For this review, take the finished solid that the model builds, in its own axes (mm). A direction names the side the tool comes from. Coordinates: 2 decimals unless noted, no trailing zeros. Write each loop counter-clockwise with the first axis right and the second up, starting at its lowest first coordinate (ties: lowest second). Pieces come first, ordered by that corner, then holes.
1) Insertion check: P1, Ø2, axis at x = -11.5, z = -10.5, coming from the +Y side; P2, Ø10, axis at x = -7.5, y = 46.5, coming from the +Z side; P3, Ø9, axis at x = -10.5, z = 11, coming from the -Y side. Each pin has a flat end and moves straight along its axis. Give the tip position at first contact, or say it passes through.
2) Mouldability with a two-part tool opening along X and no side actions: class faces 1 (the face through (-6.55, 46.07, 5.19)), 2 (the face through (9, 10, 9)), 3 (the face through (-4, 0, -4)), 4 (the face through (15.244, 50.75, -2.002)) as pulls with the +X half, pulls with the -X half, needs draft (parallel to the pull), parting line crosses it, or undercut.
3) For faces 5 (the face through (-7, 41, 4)), 6 (the face through (0, 5, -11)), 7 (the face through (0, 58, 0)), list the 3-axis set-ups (+Z, -Z, +X, -X, +Y, -Y) from which the entire face can be reached by the end or side of a thin tool; tool diameter is ignored.
4) We need section A-A on y = 16.5. Write out the cut boundary in (x, z).
5) To check wall thickness, follow line 1 along X through (y, z) = (6, 0); line 2 along X through (y, z) = (7.75, 0); line 3 along Z through (x, y) = (12, 5). State the ranges of each line that lie inside material, in increasing order.
from build123d import *

# Parameters (mm, degrees)
SKETCH1_R           = 17.5
BOSS_EXTRUDE1_DEPTH = 10
SKETCH2_R           = 21
BOSS_EXTRUDE2_DEPTH = 37
SKETCH3_R           = 15
BOSS_EXTRUDE3_DEPTH = 4
SKETCH4_R           = 5.5
BOSS_EXTRUDE4_DEPTH = 7
SKETCH5_R           = 2.5
BOSS_EXTRUDE5_DEPTH = 21
SKETCH6_R           = 1.5
SKETCH6_R_2         = 4
CUT_EXTRUDE1_DEPTH  = 10
SKETCH7_R           = 5.25
BOSS_EXTRUDE6_DEPTH = 6.5
SKETCH9_R           = 1.25
CUT_EXTRUDE2_DEPTH  = 10


with BuildPart() as part:
    # Sketch1 → Boss-Extrude1 (new body)
    with BuildSketch(Plane(origin=(0, 0, 0), x_dir=(1, 0, 0), z_dir=(0, 1, 0))):
        with Locations(Location((0, 0, 0), (0, 0, 270))):
            Circle(SKETCH1_R)
    extrude(amount=BOSS_EXTRUDE1_DEPTH)

    # Sketch2 → Boss-Extrude2 (add)
    with BuildSketch(Plane(origin=(0, 10, 0), x_dir=(1, 0, 0), z_dir=(0, 1, 0))):
        with Locations(Location((0, 0, 0), (0, 0, 270))):
            Circle(SKETCH2_R)
    extrude(amount=BOSS_EXTRUDE2_DEPTH)

    # Sketch3 → Boss-Extrude3 (add)
    with BuildSketch(Plane(origin=(0, 47, 0), x_dir=(1, 0, 0), z_dir=(0, 1, 0))):
        with Locations(Location((0, 0, 0), (0, 0, 270))):
            Circle(SKETCH3_R)
    extrude(amount=BOSS_EXTRUDE3_DEPTH)

    # Sketch4 → Boss-Extrude4 (add)
    with BuildSketch(Plane(origin=(0, 51, 0), x_dir=(1, 0, 0), z_dir=(0, 1, 0))):
        with Locations(Location((0, 0, 0), (0, 0, 270))):
            Circle(SKETCH4_R)
    extrude(amount=BOSS_EXTRUDE4_DEPTH)

    # Sketch5 → Boss-Extrude5 (add)
    with BuildSketch(Plane.XZ):
        with Locations(Location((0, 0, 0), (0, 0, 90))):
            Circle(SKETCH5_R)
    extrude(amount=BOSS_EXTRUDE5_DEPTH)

    # loft up to a face of the part (loft1)
    loft([Face(Wire([part.edges().sort_by_distance((-12.75695098, 0, -11.979574354))[0]])), Face(Wire([part.edges().sort_by_distance((-15.308341176, 10, -14.375489225))[0]]))])

    # loft up to a face of the part (loft2)
    loft([Face(Wire([part.edges().sort_by_distance((10.934529411, 51, -10.268206589))[0]])), Face(Wire([part.edges().sort_by_distance((15.308341176, 47, -14.375489225))[0]]))])

    # Sketch6 → Cut-Extrude1 (cut)
    with BuildSketch(Plane.XZ):
        with Locations(Location((0, 12.5, 0), (0, 0, 270))):
            Circle(SKETCH6_R)
        with Locations(Location((12.5, 0, 0), (0, 0, 270))):
            Circle(SKETCH6_R)
        with Locations(Location((0, -12.5, 0), (0, 0, 270))):
            Circle(SKETCH6_R)
        with Locations(Location((-12.5, 0, 0), (0, 0, 270))):
            Circle(SKETCH6_R)
        with Locations(Location((-8.838834765, 8.838834765, 0), (0, 0, 270))):
            Circle(SKETCH6_R_2)
        with Locations(Location((8.838834765, 8.838834765, 0), (0, 0, 270))):
            Circle(SKETCH6_R_2)
        with Locations(Location((8.838834765, -8.838834765, 0), (0, 0, 270))):
            Circle(SKETCH6_R_2)
        with Locations(Location((-8.838834765, -8.838834765, 0), (0, 0, 270))):
            Circle(SKETCH6_R_2)
    extrude(amount=-CUT_EXTRUDE1_DEPTH, mode=Mode.SUBTRACT)

    # Sketch7 → Boss-Extrude6 (add)
    with BuildSketch(Plane.XZ):
        with Locations(Location((0, 0, 0), (0, 0, 90))):
            Circle(SKETCH7_R)
    extrude(amount=BOSS_EXTRUDE6_DEPTH)

    # Sketch9 → Cut-Extrude2 (cut)
    with BuildSketch(Plane(origin=(0, 51, 0), x_dir=(1, 0, 0), z_dir=(0, 1, 0))):
        with Locations(Location((0, 8, 0), (0, 0, 270))):
            Circle(SKETCH9_R)
        with Locations(Location((6.92820323, -4, 0), (0, 0, 270))):
            Circle(SKETCH9_R)
        with Locations(Location((-6.92820323, -4, 0), (0, 0, 270))):
            Circle(SKETCH9_R)
    extrude(amount=-CUT_EXTRUDE2_DEPTH, mode=Mode.SUBTRACT)


solid = part.part
Result:
1. P1: stops at y = 51
1. P2: stops at z = 20.85
1. P3: stops at y = 0
2. face 1: undercut
2. face 2: undercut
2. face 3: needs draft
2. face 4: parting line crosses it
3. face 5: +Y
3. face 6: -Y
3. face 7: +Z, -Z, +X, -X, +Y
4. outline: circle Ø42 at (0, 0)
5. line 1: x = -19.6 to -14, -11 to 11, 14 to 19.6
5. line 2: x = -20.21 to -14, -11 to 11, 14 to 20.21
5. line 3: z = -15.05 to -11.29, -6.39 to -1.41, 1.41 to 6.39, 11.29 to 15.05
